from build123d import *

# Parameters (mm, degrees)
SKETCH1_W           = 150
SKETCH1_H           = 57.32
BOSS_EXTRUDE1_DEPTH = 7.5
SKETCH2_R           = 5.1
BOSS_EXTRUDE2_DEPTH = 17.5
FILLET1_R           = 5
SKETCH3_R           = 3.6
CUT_EXTRUDE1_DEPTH  = 25
SKETCH4_W           = 30
SKETCH4_H           = 7.5
CUT_EXTRUDE2_DEPTH  = 13.75
CHAMFER1_SIZE       = 5
SKETCH5_W           = 80
SKETCH5_H           = 7.5
BOSS_EXTRUDE3_DEPTH = 10.5
CHAMFER2_SIZE       = 5
SKETCH6_R           = 1.5
CUT_EXTRUDE3_DEPTH  = 7.5
SKETCH11_W          = 150
SKETCH11_H          = 7.5
BOSS_EXTRUDE5_DEPTH = 14.5
CHAMFER3_SIZE       = 5
SKETCH12_W          = 25
SKETCH12_H          = 4
BOSS_EXTRUDE6_DEPTH = 25
SKETCH13_W          = 25
SKETCH13_H          = 18.6
CUT_EXTRUDE4_DEPTH  = 7.5
SKETCH14_R          = 1.5
CUT_EXTRUDE5_DEPTH  = 4
FILLET2_R           = 2.5


with BuildPart() as part:
    # Sketch1 → Boss-Extrude1 (new body)
    with BuildSketch(Plane(origin=(0, 0, 0), x_dir=(1, 0, 0), z_dir=(0, 1, 0))):
        Rectangle(SKETCH1_W, SKETCH1_H)
    extrude(amount=BOSS_EXTRUDE1_DEPTH)

    # Sketch2 → Boss-Extrude2 (add)
    with BuildSketch(Plane(origin=(0, 7.5, 0), x_dir=(1, 0, 0), z_dir=(0, 1, 0))):
        with Locations(Location((-45, 0, 0), (0, 0, 270))):
            Circle(SKETCH2_R)
        with Locations(Location((45, 0, 0), (0, 0, 270))):
            Circle(SKETCH2_R)
    extrude(amount=BOSS_EXTRUDE2_DEPTH)

    # Fillet1
    fillet1_edges = [part.edges().sort_by_distance(p)[0] for p in [
        (-45, 7.5, -5.1),
        (45, 7.5, -5.1),
    ]]
    fillet(fillet1_edges, radius=FILLET1_R)

    # Sketch3 → Cut-Extrude1 (cut)
    with BuildSketch(Plane(origin=(0, 25, 0), x_dir=(1, 0, 0), z_dir=(0, 1, 0))):
        with Locations(Location((-45, 0, 0), (0, 0, 270))):
            Circle(SKETCH3_R)
        with Locations(Location((45, 0, 0), (0, 0, 270))):
            Circle(SKETCH3_R)
    extrude(amount=-CUT_EXTRUDE1_DEPTH, mode=Mode.SUBTRACT)

    # Sketch4 → Cut-Extrude2 (cut)
    with BuildSketch(Plane(origin=(0, 0, -28.66), x_dir=(-1, 0, 0), z_dir=(0, 0, -1))):
        with Locations((-60, 3.75)):
            Rectangle(SKETCH4_W, SKETCH4_H)
        with Locations((60, 3.75)):
            Rectangle(SKETCH4_W, SKETCH4_H)
    extrude(amount=-CUT_EXTRUDE2_DEPTH, mode=Mode.SUBTRACT)

    # Chamfer1
    chamfer1_edges = [part.edges().sort_by_distance(p)[0] for p in [
        (75, 3.75, -14.91),
        (45, 3.75, -28.66),
        (-75, 3.75, -14.91),
        (-45, 3.75, -28.66),
    ]]
    chamfer(chamfer1_edges, length=CHAMFER1_SIZE)

    # Sketch5 → Boss-Extrude3 (add)
    with BuildSketch(Plane(origin=(0, 0, -28.66), x_dir=(-1, 0, 0), z_dir=(0, 0, -1))):
        with Locations((0, 3.75)):
            Rectangle(SKETCH5_W, SKETCH5_H)
    extrude(amount=BOSS_EXTRUDE3_DEPTH)

    # Chamfer2
    chamfer2_edges = [part.edges().sort_by_distance(p)[0] for p in [
        (40, 3.75, -39.16),
        (-40, 3.75, -39.16),
    ]]
    chamfer(chamfer2_edges, length=CHAMFER2_SIZE)

    # Sketch6 → Cut-Extrude3 (cut)
    with BuildSketch(Plane(origin=(0, 0, -39.16), x_dir=(-1, 0, 0), z_dir=(0, 0, -1))):
        with Locations((-15, 3.75)):
            Circle(SKETCH6_R)
        with Locations((15, 3.75)):
            Circle(SKETCH6_R)
    extrude(amount=-CUT_EXTRUDE3_DEPTH, mode=Mode.SUBTRACT)

    # Sketch11 → Boss-Extrude5 (add)
    with BuildSketch(Plane.XY.offset(28.66)):
        with Locations((0, 3.75)):
            Rectangle(SKETCH11_W, SKETCH11_H)
    extrude(amount=BOSS_EXTRUDE5_DEPTH)

    # Chamfer3
    chamfer3_edges = [part.edges().sort_by_distance(p)[0] for p in [
        (-75, 3.75, 43.16),
        (75, 3.75, 43.16),
    ]]
    chamfer(chamfer3_edges, length=CHAMFER3_SIZE)

    # Sketch12 → Boss-Extrude6 (add)
    with BuildSketch(Plane(origin=(0, 7.5, 0), x_dir=(1, 0, 0), z_dir=(0, 1, 0))):
        with Locations((0, -36.97)):
            Rectangle(SKETCH12_W, SKETCH12_H)
    extrude(amount=BOSS_EXTRUDE6_DEPTH)

    # Sketch13 → Cut-Extrude4 (cut)
    with BuildSketch(Plane(origin=(0, 7.5, 0), x_dir=(1, 0, 0), z_dir=(0, 1, 0))):
        with Locations((0, -25.67)):
            Rectangle(SKETCH13_W, SKETCH13_H)
    extrude(amount=-CUT_EXTRUDE4_DEPTH, mode=Mode.SUBTRACT)

    # Sketch14 → Cut-Extrude5 (cut)
    with BuildSketch(Plane(origin=(0, 0, 34.97), x_dir=(-1, 0, 0), z_dir=(0, 0, -1))):
        with Locations((7.375, 20)):
            Circle(SKETCH14_R)
        with Locations((7.375, 27.25)):
            Circle(SKETCH14_R)
        with Locations((7.375, 12.75)):
            Circle(SKETCH14_R)
        with Locations((-7.25, 27.25)):
            Circle(SKETCH14_R)
        with Locations((0, 27.25)):
            Circle(SKETCH14_R)
        with Locations((0, 20)):
            Circle(SKETCH14_R)
        with Locations((0, 12.75)):
            Circle(SKETCH14_R)
        with Locations((-7.25, 12.75)):
            Circle(SKETCH14_R)
        with Locations((-7.25, 20)):
            Circle(SKETCH14_R)
    extrude(amount=-CUT_EXTRUDE5_DEPTH, mode=Mode.SUBTRACT)

    # Fillet2
    fillet2_edges = [part.edges().sort_by_distance(p)[0] for p in [
        (-12.5, 32.5, 36.97),
        (12.5, 32.5, 36.97),
    ]]
    fillet(fillet2_edges, radius=FILLET2_R)


solid = part.part
Check sheet for the modelled part. Datum: model origin and axes. Units: mm. A direction names the side the tool comes from. Round coordinates to 2 decimals unless told otherwise and drop trailing zeros. Loops run counter-clockwise (first coordinate to the right, second up) from the corner with the lowest first, then second, coordinate; pieces in that order, holes last. Notation, with made-up numbers: (41.25, 71.5) -> (86.25, 71.5) arc R11 ccw to (86.25, 91.5) -> close; hole circle Ø6 at (11, -33.75). An arc over 180 degrees is marked (long way). Put each result on its own line as item: value. Start each with the question number.
1. Gauge pin test, flat ends, axial feed: pin 1 (2.5 mm diameter, centred on x = 0, y = 12.75, fed in from +Z); pin 2 (6 mm diameter, centred on y = 17.5, z = 0, fed in from -X); pin 3 (1.6 mm diameter, centred on y = 5.5, z = -31, fed in from +X); pin 4 (5 mm diameter, centred on x = -47.5, z = -2, fed in from +Y). Record the tip position at first contact, or that the pin passes through.
2. Scan lines: probe 1 along Y at (x, z) = (7, 37); probe 2 along X at (y, z) = (17, 0); probe 3 along X at (y, z) = (6, 19). Record each from-to range of solid material in increasing order.
3. Section check C-C (y = 3.75). Give the number of separate pieces and of enclosed holes in the cut face, plus the area to 3 significant figures.
4. Access from +Z, -Z, +X, -X, +Y, -Y to the whole of each face (thin tool, end or side, straight path). Record for faces 1 (the face through (-12.5, 19, 37)), 2 (the face through (12.5, 19, 37)), 3 (the face through (-49.5, 18.7, 2.4)), 4 (the face through (-57, 4, -14.91)).
5. Section check A-A (y = 17). Enter the section's corners in (x, z), plus the area to 3 significant figures.
6. Draft check along Y on faces 5 (the face through (-48.3, 25, 2.2)), 6 (the face through (15, 4, -31.66)), 7 (the face through (48.57, 12.68, -0.47)). Enter one of: +Y half, -Y half, draft (parallel to the pull), parting line (faces both ways), or undercut.
7. Section check B-B (x = 7.25). Enter the section's corners in (y, z), plus the area to 3 significant figures.
8. Section check D-D (y = 27.25). Enter the section's corners in (x, z) (3 decimals), plus the area to 3 significant figures.
Findings:
1. pin 1: passes through
1. pin 2: stops at x = -50.1
1. pin 3: stops at x = 40
1. pin 4: stops at y = 25
2. probe 1: y = 0 to 11.27, 14.23 to 18.52, 21.48 to 25.77, 28.73 to 32.5
2. probe 2: x = -50.1 to -48.6, -41.4 to -39.9, 39.9 to 41.4, 48.6 to 50.1
2. probe 3: x = -75 to -12.5, 12.5 to 75
3. separate pieces: 1
3. enclosed holes: 3
3. area: 10,100 mm^2
4. face 1: +Z, -Z, -X, +Y
4. face 2: +Z, -Z, +X, +Y
4. face 3: +Y
4. face 4: -Z, -X, +Y, -Y
5. outline: circle Ø10.2 at (-45, 0); (-12.5, 34.97) -> (12.5, 34.97) -> (12.5, 38.97) -> (-12.5, 38.97) -> close; circle Ø10.2 at (45, 0); hole circle Ø7.2 at (-45, 0); hole circle Ø7.2 at (45, 0)
5. area: 182 mm^2
6. face 5: +Y half
6. face 6: undercut
6. face 7: draft
7. outline: (0, -39.16) -> (7.5, -39.16) -> (7.5, 16.37) -> (0, 16.37) -> close; (0, 34.97) -> (11.25, 34.97) -> (11.25, 38.97) -> (7.5, 38.97) -> (7.5, 43.16) -> (0, 43.16) -> close; (14.25, 34.97) -> (18.5, 34.97) -> (18.5, 38.97) -> (14.25, 38.97) -> close; (21.5, 34.97) -> (25.75, 34.97) -> (25.75, 38.97) -> (21.5, 38.97) -> close; (28.75, 34.97) -> (32.5, 34.97) -> (32.5, 38.97) -> (28.75, 38.97) -> close
7. area: 542 mm^2
8. outline: (-12.5, 34.97) -> (-8.875, 34.97) -> (-8.875, 38.97) -> (-12.5, 38.97) -> close; (-5.875, 34.97) -> (-1.5, 34.97) -> (-1.5, 38.97) -> (-5.875, 38.97) -> close; (1.5, 34.97) -> (5.75, 34.97) -> (5.75, 38.97) -> (1.5, 38.97) -> close; (8.75, 34.97) -> (12.5, 34.97) -> (12.5, 38.97) -> (8.75, 38.97) -> close
8. area: 64.0 mm^2
